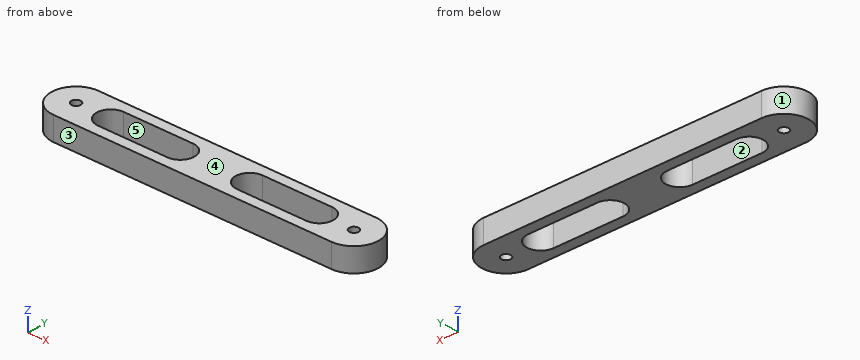
```python
from build123d import *

# Parameters (mm, degrees)
EXTRUDE_1_DEPTH     = 50
SKETCH_2_R          = 10
CUT_EXTRUDE_1_DEPTH = 657.515422515


with BuildPart() as part:
    # 草图1 → 凸台-拉伸1 (new body)
    with BuildSketch(Plane.XY):
        with BuildLine():
            Line((0, 52.5), (600, 52.5))
            ThreePointArc((600, 52.5), (652.5, 0), (600, -52.5))
            Line((600, -52.5), (0, -52.5))
            ThreePointArc((0, -52.5), (-52.5, 0), (0, 52.5))
        make_face()
    extrude(amount=EXTRUDE_1_DEPTH)

    # 草图2 → 切除-拉伸1 (cut, through all)
    with BuildSketch(Plane.XY.offset(50)):
        with BuildLine():
            Line((375, -30), (525, -30))
            ThreePointArc((525, -30), (555, 0), (525, 30))
            Line((525, 30), (375, 30))
            ThreePointArc((375, 30), (345, 0), (375, -30))
        make_face()
        with Locations((600, 0)):
            Circle(SKETCH_2_R)
        Circle(SKETCH_2_R)
        with BuildLine():
            Line((75, -30), (225, -30))
            ThreePointArc((225, -30), (255, 0), (225, 30))
            Line((225, 30), (75, 30))
            ThreePointArc((75, 30), (45, 0), (75, -30))
        make_face()
    extrude(amount=-CUT_EXTRUDE_1_DEPTH, mode=Mode.SUBTRACT)


solid = part.part
```
Input: part model. Units: mm. Frame: model coordinates. Face numbers are marked on the shaded views. A direction names the side the tool comes from. Give positions to 0.01 mm unless a question says otherwise; leave off trailing zeros. Order: outer loops, then holes, each group sorted by start corner. A loop starts at its lowest first (then second) coordinate and runs counter-clockwise, first axis right, second up. Notation, with made-up numbers: M -29.75,79.25 L -14.75,79.25 A19 cw -14.75,89.25 Z; hole C 88,70.25 d10. An arc over 180 degrees is marked long. Return JSON: item names as keys, results as strings.
1) Section query B-B on x = 162. Output: boundary loops of the cut face in (y, z).
Taken from the geometry:
{"outline": "M -52.5,0 L -30,0 L -30,50 L -52.5,50 Z; M 30,0 L 52.5,0 L 52.5,50 L 30,50 Z"}
2) Line query: L1, parallel to Y at x = 0, z = 15.5; L2, parallel to Y at x = 504.5, z = 9; L3, parallel to X at y = -4, z = 16. Output: solid intervals per line, ascending. Write a range as [from, to].
Taken from the geometry:
{"L1": "y = [-52.5, -10], [10, 52.5]", "L2": "y = [-52.5, -30], [30, 52.5]", "L3": "x = [-52.35, -9.17], [9.17, 45.27], [254.73, 345.27], [554.73, 590.83], [609.17, 652.35]"}
3) Mould query, pull axis Y, two halves, no side actions, for the marked faces 1, 2 and 3. Classes: released by +Y, released by -Y, zero draft, split by the parting line, or undercut.
Taken from the geometry:
{"face 1": "split by the parting line", "face 2": "undercut", "face 3": "released by -Y"}
4) Access query for the marked faces 4 and 5. Directions: +Z, -Z, +X, -X, +Y, -Y. A direction counts if a zero-diameter tool reaches every point of the face in a straight line with its end or side. Return the directions, or none.
Taken from the geometry:
{"face 4": "+Z, +X, -X, +Y, -Y", "face 5": "+Z, -Z"}
5) Section query D-D on x = 541. Output: boundary loops of the cut face in (y, z).
Taken from the geometry:
{"outline": "M -52.5,0 L -25.38,0 L -25.38,50 L -52.5,50 Z; M 25.38,0 L 52.5,0 L 52.5,50 L 25.38,50 Z"}
6) Contact query for flat-ended pins moving along their axis: pin 1 (1 mm diameter, centred on y = -28, z = 7, fed in from -X); pin 2 (4 mm diameter, centred on y = 25.5, z = 27.5, fed in from -X); pin 3 (3 mm diameter, centred on y = -6, z = 9, fed in from -X). Output: stop coordinate, or through.
Taken from the geometry:
{"pin 1": "stops at x = -44.72", "pin 2": "stops at x = -46.95", "pin 3": "stops at x = -52.31"}
7) Section query C-C on z = 40.5. Output: boundary loops of the cut face in (x, y).
Taken from the geometry:
{"outline": "M 0,-52.5 L 600,-52.5 A52.5 ccw 600,52.5 L 0,52.5 A52.5 ccw Z; hole C 0,0 d20; hole M 75,-30 L 225,-30 A30 ccw 225,30 L 75,30 A30 ccw Z; hole M 375,-30 L 525,-30 A30 ccw 525,30 L 375,30 A30 ccw Z; hole C 600,0 d20"}
8) Section query A-A on y = 0. Output: boundary loops of the cut face in (x, z).
Taken from the geometry:
{"outline": "M -52.5,0 L -10,0 L -10,50 L -52.5,50 Z; M 10,0 L 45,0 L 45,50 L 10,50 Z; M 255,0 L 345,0 L 345,50 L 255,50 Z; M 555,0 L 590,0 L 590,50 L 555,50 Z; M 610,0 L 652.5,0 L 652.5,50 L 610,50 Z"}
